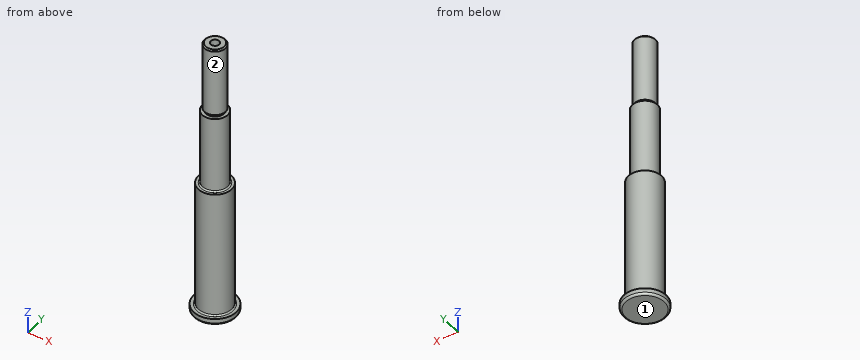
```python
from build123d import *

# Parameters (mm, degrees)
SKETCH3_R          = 3.2
CUT_EXTRUDE1_DEPTH = 35


with BuildPart() as part:
    # Sketch2 → Base-Revolve (revolve)
    with BuildSketch(Plane(origin=(0, 0, 0), x_dir=(0, 0, -1), z_dir=(1, 0, 0)), mode=Mode.PRIVATE) as base_revolve_sk:
        with BuildLine():
            Line((0, 0), (0, 14.4))
            ThreePointArc((0, 14.4), (-0.439339828, 15.460660172), (-1.5, 15.9))
            Line((-1.5, 15.9), (-4.6, 15.9))
            Line((-4.6, 15.9), (-4.6, 13.5))
            ThreePointArc((-4.6, 13.5), (-4.892893219, 12.792893219), (-5.6, 12.5))
            Line((-5.6, 12.5), (-99.9, 12.5))
            Line((-99.9, 12.5), (-99.9, 10.5))
            ThreePointArc((-99.9, 10.5), (-100.192893219, 9.792893219), (-100.9, 9.5))
            Line((-100.9, 9.5), (-157.1, 9.5))
            Line((-157.1, 9.5), (-157.1, 6.85))
            Line((-157.1, 6.85), (-159.1, 6.85))
            Line((-159.1, 6.85), (-159.1, 7.95))
            Line((-159.1, 7.95), (-209, 7.95))
            Line((-209, 7.95), (-210, 6.95))
            Line((-210, 6.95), (-210, 0))
            Line((-210, 0), (0, 0))
        make_face()
    revolve(base_revolve_sk.sketch.rotate(Axis((0, 0, 0), (0, 0, -1)), 90), axis=Axis((0, 0, 0), (0, 0, -1)))

    # Sketch3 → Cut-Extrude1 (cut)
    with BuildSketch(Plane.XY.offset(210)):
        Circle(SKETCH3_R)
    extrude(amount=-CUT_EXTRUDE1_DEPTH, mode=Mode.SUBTRACT)


solid = part.part
```
The model under review builds one solid part; all positions refer to its coordinate system, in mm. Face numbers are marked on the shaded views. A direction names the side the tool comes from. Round coordinates to 2 decimals unless told otherwise and drop trailing zeros. Loops run counter-clockwise (first coordinate to the right, second up) from the corner with the lowest first, then second, coordinate; pieces in that order, holes last.
1) Tool access review of the marked faces 1 and 2: name each direction out of +Z, -Z, +X, -X, +Y, -Y from which nothing blocks a thin tool from reaching the whole face with its end or side.
Values follow:
face 1: -Z, +X, -X, +Y, -Y
face 2: +Z
2) Consider section D-D on z = 163. State the section outline as (x, y) points.
Values follow:
outline: circle Ø15.9 at (0, 0)
3) Consider section C-C on z = 33.5. State the section outline as (x, y) points, then the cut area to 3 significant figures.
Values follow:
outline: circle Ø25 at (0, 0)
area: 491 mm2
4) Wall thickness on line 1 along Y through (x, z) = (0, 201); line 2 along Z through (x, y) = (-7.5, -11); line 3 along Z through (x, y) = (-11.5, 2): over which ranges is each line inside the solid? List them lowest first.
Values follow:
line 1: y = -7.95 to -3.2, 3.2 to 7.95
line 2: z = 0 to 4.62
line 3: z = 0 to 99.9
5) Clearance check with flat-ended pins moving along their axes: P1, Ø1.5, axis at x = 4, z = 48, coming from the -Y side; P2, Ø5, axis at x = -9, y = 8.5, coming from the +Z side; P3, Ø2, axis at y = -8, z = 137.5, coming from the -X side. State where each tip first meets the part, or that it passes through.
Values follow:
P1: stops at y = -12.07
P2: stops at z = 100.12
P3: stops at x = -6.42
